```python
from build123d import *

# Parameters (mm, degrees)
SKETCH1_R           = 4.5
BOSS_EXTRUDE1_DEPTH = 3
SKETCH2_R           = 5.15
BOSS_EXTRUDE2_DEPTH = 1
SKETCH3_R           = 2
CUT_EXTRUDE1_DEPTH  = 9.309332103
SKETCH4_R           = 4.05
SKETCH4_R_2         = 2.6
CUT_EXTRUDE2_DEPTH  = 0.06
CUT_EXTRUDE3_START  = -0.06
SKETCH5_R           = 4.05
SKETCH5_R_2         = 2.6
CUT_EXTRUDE3_DEPTH  = 0.06
FILLET1_R           = 0.15


with BuildPart() as part:
    # Sketch1 → Boss-Extrude1 (new body)
    with BuildSketch(Plane.XY):
        Circle(SKETCH1_R)
    extrude(amount=BOSS_EXTRUDE1_DEPTH)

    # Sketch2 → Boss-Extrude2 (add)
    with BuildSketch(Plane.XY.offset(3)):
        Circle(SKETCH2_R)
    extrude(amount=BOSS_EXTRUDE2_DEPTH)

    # Sketch3 → Cut-Extrude1 (cut, through all)
    with BuildSketch(Plane.XY.offset(4)):
        Circle(SKETCH3_R)
    extrude(amount=-CUT_EXTRUDE1_DEPTH, mode=Mode.SUBTRACT)

    # Sketch4 → Cut-Extrude2 (cut)
    with BuildSketch(Plane.XY.offset(4)):
        Circle(SKETCH4_R)
        Circle(SKETCH4_R_2, mode=Mode.SUBTRACT)
    extrude(amount=-CUT_EXTRUDE2_DEPTH, mode=Mode.SUBTRACT)

    # Sketch5 → Cut-Extrude3 (cut)
    with BuildSketch(Plane(origin=(0, 0, 0), x_dir=(-1, 0, 0), z_dir=(0, 0, -1)).offset(CUT_EXTRUDE3_START)):
        with Locations(Location((0, 0, 0), (0, 0, 180))):
            Circle(SKETCH5_R)
        with Locations(Location((0, 0, 0), (0, 0, 180))):
            Circle(SKETCH5_R_2, mode=Mode.SUBTRACT)
    extrude(amount=CUT_EXTRUDE3_DEPTH, mode=Mode.SUBTRACT)

    # Fillet1
    fillet1_edges = [part.edges().sort_by_distance(p)[0] for p in [
        (-2, 0, 0),
        (-2, 0, 4),
        (-4.5, 0, 0),
        (-5.15, 0, 4),
    ]]
    fillet(fillet1_edges, radius=FILLET1_R)


solid = part.part
```
Geometry: final body of the model. Coordinates: model frame, mm. A direction names the side the tool comes from. Round coordinates to 2 decimals unless told otherwise and drop trailing zeros. Order: outer loops, then holes, each group sorted by start corner. A loop starts at its lowest first (then second) coordinate and runs counter-clockwise, first axis right, second up. Notation, with made-up numbers: (26, -24.5) - (65, -24.5) arc R26 ccw to (65, 14.5) - close; hole circle Ø7 at (3, 63.5). An arc over 180 degrees is marked (long way). Use CSV: the item, a comma, the result in double quotes. Start each with the question number.
Q1. Section query A-A (z = 2.35). Return loops of the section in (x, y).
Q2. First-contact query: pin 1 (1.5 mm diameter, centred on x = -4, y = 2, fed in from -Z); pin 2 (1.5 mm diameter, centred on x = -3, z = 2.5, fed in from +Y). Flat tips, straight axial feed; report the tip coordinate or a pass-through.
Q3. Mould query, pull axis X, two halves, no side actions, for faces 3 (the face through (3, 0, 0.06)), 4 (the face through (-0.59, 4.46, 1.56)), 5 (the face through (0, -5, 3)). Classes: +X half, -X half, draft (parallel to the pull), parting line (faces both ways), or undercut.
Q4. Access query for faces 1 (the face through (2, -4, 4)), 2 (the face through (0, -3, 3.94)). Directions: +Z, -Z, +X, -X, +Y, -Y. A direction counts if a zero-diameter tool reaches every point of the face in a straight line with its end or side. Return the directions, or none.
Q5. Material intervals for line 1 along Z through (x, y) = (-3.25, -3.25); line 2 along X through (y, z) = (-1.25, 0.25); line 3 along Z through (x, y) = (0.5, 3.25), sorted ascending. Write a range as from..to.
Q6. Section query B-B (z = 3.7). Return loops of the section in (x, y), and give its area (3 significant figures).
Result set:
1,outline,"circle Ø9 at (0, 0); hole circle Ø4 at (0, 0)"
2,pin 1,"stops at z = 0"
2,pin 2,"stops at y = 4.53"
3,face 3,"undercut"
3,face 4,"parting line"
3,face 5,"draft"
4,face 1,"+Z, +X, -X, +Y, -Y"
4,face 2,"+Z"
5,line 1,"z = 3..4"
5,line 2,"x = -4.32..-1.56, 1.56..4.32"
5,line 3,"z = 0.06..3.94"
6,outline,"circle Ø10.3 at (0, 0); hole circle Ø4 at (0, 0)"
6,area,"70.8 mm2"
